```python
from build123d import *

# Parameters (mm, degrees)
SCHIZZO2_W                   = 42
SCHIZZO2_H                   = 42
ESTRUSIONE_ESTRUSIONE1_DEPTH = 12
SCHIZZO3_R                   = 11
TAGLIO_ESTRUSIONE1_DEPTH     = 12
TAGLIO_ESTRUSIONE2_DEPTH     = 42
SMUSSO2_SIZE                 = 2
SMUSSO3_SIZE                 = 2
SMUSSO4_SIZE                 = 2
SMUSSO5_SIZE                 = 2


with BuildPart() as part:
    # Schizzo2 → Estrusione-Estrusione1 (new body)
    with BuildSketch(Plane.XY):
        Rectangle(SCHIZZO2_W, SCHIZZO2_H)
    extrude(amount=ESTRUSIONE_ESTRUSIONE1_DEPTH)

    # Schizzo3 → Taglio-Estrusione1 (cut)
    with BuildSketch(Plane.XY):
        Circle(SCHIZZO3_R)
    extrude(amount=TAGLIO_ESTRUSIONE1_DEPTH, mode=Mode.SUBTRACT)

    # Schizzo5 → Taglio-Estrusione2 (cut)
    with BuildSketch(Plane(origin=(21, 0, 0), x_dir=(0, 0, -1), z_dir=(1, 0, 0))):
        with BuildLine():
            Line((-1.976058117, 11.770215969), (-1.976058117, -11.829784031))
            ThreePointArc((-1.976058117, -11.829784031), (-5.976058117, -15.829784031), (-9.976058117, -11.829784031))
            Line((-9.976058117, -11.829784031), (-9.976058117, 11.770215969))
            ThreePointArc((-9.976058117, 11.770215969), (-5.976058117, 15.770215969), (-1.976058117, 11.770215969))
        make_face()
    extrude(amount=-TAGLIO_ESTRUSIONE2_DEPTH, mode=Mode.SUBTRACT)

    # Smusso2
    smusso2_edges = [part.edges().sort_by_distance(p)[0] for p in [
        (-21, 21, 6),
    ]]
    chamfer(smusso2_edges, length=SMUSSO2_SIZE)

    # Smusso3
    smusso3_edges = [part.edges().sort_by_distance(p)[0] for p in [
        (21, 21, 6),
    ]]
    chamfer(smusso3_edges, length=SMUSSO3_SIZE)

    # Smusso4
    smusso4_edges = [part.edges().sort_by_distance(p)[0] for p in [
        (21, -21, 6),
    ]]
    chamfer(smusso4_edges, length=SMUSSO4_SIZE)

    # Smusso5
    smusso5_edges = [part.edges().sort_by_distance(p)[0] for p in [
        (-21, -21, 6),
    ]]
    chamfer(smusso5_edges, length=SMUSSO5_SIZE)


solid = part.part
```
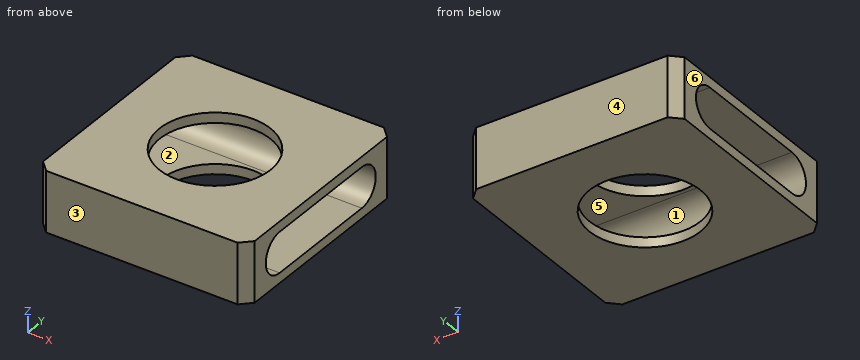
Verification items for the finished model (mm, model axes). Face numbers are marked on the shaded views. A direction names the side the tool comes from. Give positions to 0.01 mm unless a question says otherwise; leave off trailing zeros. Order: outer loops, then holes, each group sorted by start corner. A loop starts at its lowest first (then second) coordinate and runs counter-clockwise, first axis right, second up. Notation, with made-up numbers: M 41,3 L 72,3 A31 ccw 72,38 Z; hole C 61.25,75.25 d2. An arc over 180 degrees is marked long. Answer in a Markdown table with one row per item. Add a question column.
Item 1: Section check A-A, the plane x = 0. Enter the section's corners in (y, z).
Item 2: Mould release check, pull along Y, two halves, no side actions. Record for the marked faces 1, 2, 3 and 4: released by +Y, released by -Y, zero draft, split by the parting line, or undercut.
Item 3: Tool access check on the marked faces 5 and 6. Record the directions out of +Z, -Z, +X, -X, +Y, -Y that give a thin tool (end or side, any length) a straight path to the whole face; none if there is none.
Item 4: Section check C-C, the plane z = 7.75. Enter the section's corners in (x, y).
Item 5: Section check D-D, the plane z = 1.25. Enter the section's corners in (x, y), and give its area (3 significant figures).
Item 6: Section check B-B, the plane y = 0. Enter the section's corners in (x, z).
Item 7: Scan lines: probe 1 along Y at (x, z) = (0, 0.45); probe 2 along Z at (x, y) = (17, -4). Record each from-to range of solid material in increasing order. Write a range as from..to.
Filled sheet:
| question | item | result |
|---|---|---|
| 1 | outline | M -21,0 L -11,0 L -11,1.98 L -11.83,1.98 A4 cw -11.83,9.98 L -11,9.98 L -11,12 L -21,12 Z; M 11,0 L 21,0 L 21,12 L 11,12 L 11,9.98 L 11.77,9.98 A4 cw 11.77,1.98 L 11,1.98 Z |
| 2 | face 1 | undercut |
| 2 | face 2 | undercut |
| 2 | face 3 | released by -Y |
| 2 | face 4 | released by +Y |
| 3 | face 5 | +X, -X |
| 3 | face 6 | +Z, -Z, -X, +Y, -Y |
| 4 | outline | M -21,-19 L -19,-21 L 19,-21 L 21,-19 L 21,-15.41 L -21,-15.41 Z; M -21,15.36 L 21,15.36 L 21,19 L 19,21 L -19,21 L -21,19 Z |
| 5 | outline | M -21,-19 L -19,-21 L 19,-21 L 21,-19 L 21,19 L 19,21 L -19,21 L -21,19 Z; hole C 0,0 d22 |
| 5 | area | 1,380 mm^2 |
| 6 | outline | M -21,0 L -11,0 L -11,1.98 L -21,1.98 Z; M -21,9.98 L -11,9.98 L -11,12 L -21,12 Z; M 11,0 L 21,0 L 21,1.98 L 11,1.98 Z; M 11,9.98 L 21,9.98 L 21,12 L 11,12 Z |
| 7 | probe 1 | y = -21..-11, 11..21 |
| 7 | probe 2 | z = 0..1.98, 9.98..12 |
